from build123d import *

# Parameters (mm, degrees)
BOX001001011_W     = 120
BOX001001011_H     = 80
BOX001001011_DEPTH = 12
FILLET003002007_R  = 20
FILLET003002008_R  = 20
FILLET003002009_R  = 6
FILLET003002010_R  = 2
FILLET003002011_R  = 5.5


with BuildPart() as part:
    # Box001001011 → Box001001011 (new body)
    with BuildSketch(Plane(origin=(39, -40, 73), x_dir=(1, 0, 0), z_dir=(0, 0, 1))):
        with Locations((60, 40)):
            Rectangle(BOX001001011_W, BOX001001011_H)
    extrude(amount=BOX001001011_DEPTH)

    # Fillet003002007
    fillet003002007_edges = [part.edges().sort_by_distance(p)[0] for p in [
        (159, -40, 79),
    ]]
    fillet(fillet003002007_edges, radius=FILLET003002007_R)

    # Fillet003002008
    fillet003002008_edges = [part.edges().sort_by_distance(p)[0] for p in [
        (159, 40, 79),
    ]]
    fillet(fillet003002008_edges, radius=FILLET003002008_R)

    # Fillet003002009
    fillet003002009_edges = [part.edges().sort_by_distance(p)[0] for p in [
        (39, 0, 73),
    ]]
    fillet(fillet003002009_edges, radius=FILLET003002009_R)

    # Fillet003002010
    fillet003002010_edges = [part.edges().sort_by_distance(p)[0] for p in [
        (89, 40, 85),
    ]]
    fillet(fillet003002010_edges, radius=FILLET003002010_R)

    # Fillet003002011
    fillet003002011_edges = [part.edges().sort_by_distance(p)[0] for p in [
        (39, 0, 85),
    ]]
    fillet(fillet003002011_edges, radius=FILLET003002011_R)


solid = part.part
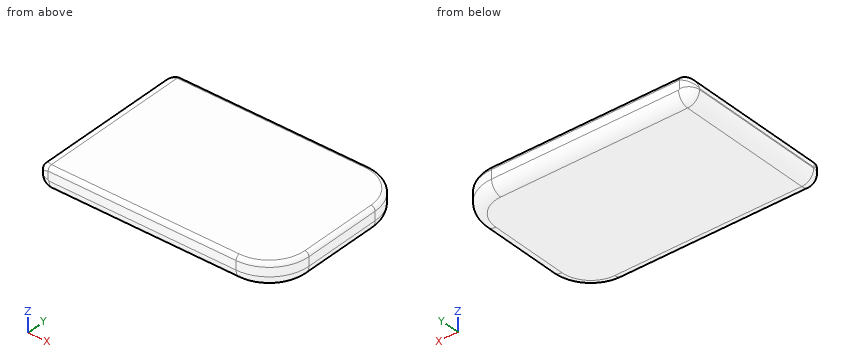
The listing builds one solid part. Answer for the finished solid, in the listing's coordinates (mm). Coordinates: 2 decimals unless noted, no trailing zeros. Order: outer loops, then holes, each group sorted by start corner. A loop starts at its lowest first (then second) coordinate and runs counter-clockwise, first axis right, second up. Notation, with made-up numbers: (41.25, 72.5) -> (51.25, 72.5) arc R26 ccw to (51.25, 86.5) -> close; hole circle Ø4 at (-4.5, -9). An arc over 180 degrees is marked (long way). Answer in a Markdown table with one row per item. Add a question column.
Item 1: Find the intervals of material crossed by L1, parallel to Y at x = 140, z = 83; L2, parallel to X at y = -17, z = 79.75; L3, parallel to X at y = 26, z = 79.5, in increasing order. Write a range as from..to.
Item 2: Find section A-A (x = 112.5). Write down the section's boundary in (y, z).
Item 3: This flat-tipped pin is pushed along its axis until it touches: P1, Ø3, axis at y = 23, z = 83.5, coming from the +X side. Where does it stop, or does it pass through?
Result set:
| question | item | result |
|---|---|---|
| 1 | L1 | y = -39.97..39.97 |
| 1 | L2 | x = 39.01..159 |
| 1 | L3 | x = 39..158.08 |
| 2 | outline | (-40, 78.5) arc R5.5 ccw to (-34.5, 73) -> (34.5, 73) arc R5.5 ccw to (40, 78.5) -> (40, 83) arc R2 ccw to (38, 85) -> (-38, 85) arc R2 ccw to (-40, 83) -> close |
| 3 | P1 | stops at x = 158.94 |
